from build123d import *

# Parameters (mm, degrees)
SKETCH1_R           = 1.75
BOSS_EXTRUDE1_DEPTH = 3


with BuildPart() as part:
    # Sketch1 → Boss-Extrude1 (new body)
    with BuildSketch(Plane.XY):
        with BuildLine():
            Line((19.930411003, 2.905988798), (13.87145238, 1.735459786))
            ThreePointArc((13.87145238, 1.735459786), (11.531557717, 1.972597442), (9.296030987, 2.703187301))
            ThreePointArc((9.296030987, 2.703187301), (3.919484189, 8.419131518), (4.006841218, 16.265891519))
            ThreePointArc((4.006841218, 16.265891519), (1.723665713, 17.781070836), (-0.941946899, 18.416026075))
            ThreePointArc((-0.941946899, 18.416026075), (-1.568863415, 18.470126635), (-2.197160171, 18.50468636))
            ThreePointArc((-2.197160171, 18.50468636), (-5.87970066, 13.635417111), (-8.639038917, 8.189598545))
            ThreePointArc((-8.639038917, 8.189598545), (-8.697179287, 6.801867653), (-8.727525387, 5.413250916))
            ThreePointArc((-8.727525387, 5.413250916), (-8.707936379, 5.106364202), (-8.683372389, 4.799835582))
            add(Edge.make_bspline(
                [(-8.683372389, 4.799835582), (-8.588074591, 3.721163805), (-8.402294299, 2.674479561), (-7.859371187, 0.648508115), (-7.502052979, -0.331606117), (-7.064007696, -1.28129998)],
                knots=[0, 0, 0, 0, 0.5, 0.5, 1, 1, 1, 1], degree=3))
            add(Edge.make_bspline(
                [(-7.064007696, -1.28129998), (-6.575170871, -2.34111126), (-5.98506043, -3.361216675), (-4.957629948, -4.84262589), (-4.59187789, -5.329143335), (-3.817976232, -6.281801183), (-3.40882724, -6.74810305), (-2.97381792, -7.203826342)],
                knots=[0, 0, 0, 0, 0.5, 0.5, 0.75, 0.75, 1, 1, 1, 1], degree=3))
            add(Edge.make_bspline(
                [(-2.97381792, -7.203826342), (-2.306446509, -7.902976179), (-1.590279206, -8.56570689), (-0.445412997, -9.35234524), (-0.053513063, -9.579507747), (0.556953087, -9.853650755), (0.764136141, -9.933887283), (1.181773294, -10.067725648), (1.391009263, -10.121047129), (1.602766598, -10.159905725)],
                knots=[0, 0, 0, 0, 0.5, 0.5, 0.75, 0.75, 0.875, 0.875, 1, 1, 1, 1], degree=3))
            add(Edge.make_bspline(
                [(1.602766598, -10.159905725), (2.019871783, -10.236446742), (2.459018956, -10.260016432), (3.337272754, -10.220368292), (3.779944348, -10.157384511), (4.227454337, -10.064224837)],
                knots=[0, 0, 0, 0, 0.5, 0.5, 1, 1, 1, 1], degree=3))
            add(Edge.make_bspline(
                [(4.227454337, -10.064224837), (5.089770185, -9.88471362), (5.962802505, -9.592227299), (6.811456082, -9.284683988)],
                knots=[0, 0, 0, 0, 1, 1, 1, 1], degree=3))
            add(Edge.make_bspline(
                [(6.811456082, -9.284683988), (7.056520313, -9.195875236), (7.297794582, -9.106311657), (7.776758126, -8.924041304), (8.015576329, -8.831105295), (8.722360856, -8.547506225), (9.179802119, -8.35044286), (9.620286504, -8.127847225)],
                knots=[0, 0, 0, 0, 0.25, 0.25, 0.5, 0.5, 1, 1, 1, 1], degree=3))
            add(Edge.make_bspline(
                [(9.620286504, -8.127847225), (9.800382572, -8.036836964), (9.977339671, -7.94180455), (10.322866167, -7.742648629), (10.490967018, -7.638558401), (10.990123709, -7.307373872), (11.312673774, -7.064183232), (12.24261019, -6.291133214), (12.820931233, -5.712035881), (13.94631914, -4.501489979), (14.49233771, -3.8697351), (15.184900578, -3.09577571), (15.323634143, -2.942251733), (15.602122385, -2.637726794), (15.743780167, -2.483440537), (16.029801415, -2.186068127), (16.169367003, -2.0474533), (16.479304052, -1.785805781), (16.652919268, -1.664467301), (16.828175246, -1.561356406)],
                knots=[0, 0, 0, 0, 0.0625, 0.0625, 0.125, 0.125, 0.25, 0.25, 0.5, 0.5, 0.75, 0.75, 0.8125, 0.8125, 0.875, 0.875, 0.9375, 0.9375, 1, 1, 1, 1], degree=3))
            ThreePointArc((16.828175246, -1.561356406), (20.244272985, -0.189669108), (23.736412446, 0.974895959))
            Line((23.736412446, 0.974895959), (23.351331305, 1.380731944))
            ThreePointArc((23.351331305, 1.380731944), (23.035702836, 1.68776393), (22.696524646, 1.968563017))
            ThreePointArc((22.696524646, 1.968563017), (22.121114049, 2.363611886), (21.509254361, 2.699452157))
            ThreePointArc((21.509254361, 2.699452157), (20.73478902, 2.91705232), (19.930411003, 2.905988798))
        make_face()
        with Locations((1.955579729, -7.60507725)):
            Circle(SKETCH1_R, mode=Mode.SUBTRACT)
    extrude(amount=BOSS_EXTRUDE1_DEPTH)


solid = part.part
The model under review builds one solid part; all positions refer to its coordinate system, in mm. A direction names the side the tool comes from. Give positions to 0.01 mm unless a question says otherwise; leave off trailing zeros. Order: outer loops, then holes, each group sorted by start corner. A loop starts at its lowest first (then second) coordinate and runs counter-clockwise, first axis right, second up. Notation, with made-up numbers: M 25,33.5 L 37,33.5 A11 cw 37,38.5 Z; hole C 73,68 d2. An arc over 180 degrees is marked long. Answer in a Markdown table with one row per item. Add a question column.
1. Machinability: for faces 4 (the flat face through (16.94, 2.33, 1.48)), 5 (the cylindrical face through (1.576, -9.313, 1.479)), which of the approach directions +Z, -Z, +X, -X, +Y, -Y give a long, thin tool a straight path to every point of the face, cutting with its end or side? Answer none if there is none.
2. Add section A-A on y = 13.5. State the section outline as (x, z) points.
3. To check wall thickness, follow line 1 along X through (y, z) = (-8.75, 2.75); line 2 along X through (y, z) = (-6, 2.45); line 3 along X through (y, z) = (-3.5, 1.6). State the ranges of each line that lie inside material, in increasing order.
4. Mouldability with a two-part tool opening along Y and no side actions: class faces 1 (the cylindrical face through (3.961, 8.314, 1.479)), 2 (the flat face through (4, 1, 3)), 3 (the cylindrical face through (-1.56, 18.47, 1.48)) as released by +Y, released by -Y, zero draft, split by the parting line, or undercut.
The answers:
| question | item | result |
|---|---|---|
| 1 | face 4 | +Z, -Z, +Y |
| 1 | face 5 | +Z, -Z |
| 2 | outline | M -5.96,0 L 3.28,0 L 3.28,3 L -5.96,3 Z |
| 3 | line 1 | -1.29 to 0.63, 3.28 to 8.22 |
| 3 | line 2 | -4.05 to 1.26, 2.65 to 12.51 |
| 3 | line 3 | -5.86 to 14.82 |
| 4 | face 1 | undercut |
| 4 | face 2 | zero draft |
| 4 | face 3 | released by +Y |
